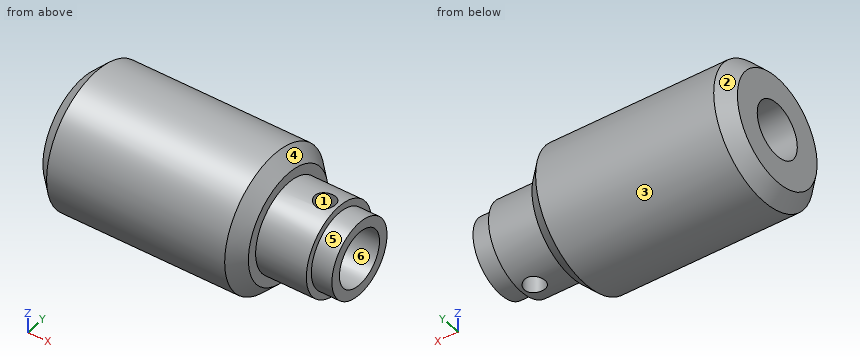
Autodesk Inventor part; units mm, degrees
ref_plane "Work Plane1" through (17.6, 0, -3.25) normal (0, 0, 1) x (1, 0, 0)
ref_plane "YZ Plane" through (0, 0, 0) normal (1, 0, 0) x (0, 1, 0)
ref_plane "XZ Plane" through (0, 0, 0) normal (0, 1, 0) x (-1, 0, 0)
sketch "Sketch1" plane through (0, 0, 0) normal (0, 0, 1) x (1, 0, 0)
  line L0 (0, 0) -> (0, 4.975)
  line L1 (0, 4.975) -> (15, 4.975)
  line L2 (15, 4.975) -> (15, 3.25)
  line L3 (15, 3.25) -> (20.2, 3.25)
  line L4 (20.2, 3.25) -> (20.2, 0)
  line L5 (20.2, 0) -> (0, 0)
  dimension "d2" = 20.2
  dimension "d3" = 15
  dimension "d19" = 9.95
  dimension "d20" = 6.5
revolve "Revolution1" add sketch "Sketch1" angle 360 about axis through (20.2, 0, 0) along (-1, 0, 0)
thread "Thread1"
chamfer "Chamfer1" distance 1 angle 45 2 edges at (15, -4.975, 0) (0, -4.975, 0)
hole "Hole1" at (20.2, 0, 0) direction (-1, 0, 0) diameter 4 end through all
ref_plane "Work Plane1" through (17.6, 0, -3.25) normal (0, 0, 1) x (1, 0, 0)
sketch "Sketch2" plane through (17.6, 0, -3.25) normal (0, 0, 1) x (1, 0, 0)
  line L0 (2.6, -3.25) -> (2.6, 3.25)
  line L1 (-2.6, -3.25) -> (-2.6, 3.25)
  point P0 (-17.6, 0)
  point P1 (0.1, 0)
  point P2 (2.6, 0)
  dimension "d21" = 2.5
hole "Hole2" at (17.7, 0, -3.25) direction (0, 0, 1) diameter 1.5 end through all
sketch "Sketch3" plane through (20.2, 0, 0) normal (1, 0, 0) x (0, 0, -1)
  circle A0 centre (0, 0) radius 2.75
  circle A1 centre (0, 0) radius 3.25
  dimension "d29" = 5.5
extrude "Extrusion1" cut sketch "Sketch3" against normal blind 1.5
properties part number "worm_1_20_conrad_with_bolt_hole" material "Steel"
Geometry: final body of the model. Coordinates: model frame, mm. Face numbers are marked on the shaded views. A direction names the side the tool comes from. Coordinates: 2 decimals unless noted, no trailing zeros. Order: outer loops, then holes, each group sorted by start corner. A loop starts at its lowest first (then second) coordinate and runs counter-clockwise, first axis right, second up.
Item 1: Access query for the marked faces 5 and 6. Directions: +Z, -Z, +X, -X, +Y, -Y. A direction counts if a zero-diameter tool reaches every point of the face in a straight line with its end or side. Return the directions, or none.
Answer:
face 5: +X
face 6: +X, -X
Item 2: Material intervals for line 1 along X through (y, z) = (0, -2.7); line 2 along Y through (x, z) = (8.75, 0) (3 decimals), sorted ascending.
Answer:
line 1: x = 0 to 16.95, 18.45 to 20.2
line 2: y = -4.975 to -2, 2 to 4.975
Item 3: Section query C-C (x = 4.75). Output: boundary loops of the cut face in (y, z) (3 decimals).
Answer:
outline: circle Ø9.95 at (0, 0); hole circle Ø4 at (0, 0)
Item 4: Section query B-B (x = 17.7). Output: boundary loops of the cut face in (y, z).
Answer:
outline: (-0.75, -3.16) - (-0.75, -1.85) arc R2 cw to (-0.75, 1.85) - (-0.75, 3.16) arc R3.25 ccw to start; (0.75, -3.16) arc R3.25 ccw to (0.75, 3.16) - (0.75, 1.85) arc R2 cw to (0.75, -1.85) - close
Item 5: Section query A-A (z = 0). Output: boundary loops of the cut face in (x, y) (3 decimals), then the cut area to 4 significant figures.
Answer:
outline: (0, -3.975) - (1, -4.975) - (14, -4.975) - (15, -3.975) - (15, -3.25) - (18.7, -3.25) - (18.7, -2.75) - (20.2, -2.75) - (20.2, -2) - (0, -2) - close; (0, 2) - (20.2, 2) - (20.2, 2.75) - (18.7, 2.75) - (18.7, 3.25) - (15, 3.25) - (15, 3.975) - (14, 4.975) - (1, 4.975) - (0, 3.975) - close
area: 98.75 mm2
Item 6: Contact query for flat-ended pins moving along their axis: P1, Ø2.5, axis at y = 0, z = 0, coming from the -X side; P2, Ø4, axis at x = 5, z = -2.5, coming from the +Y side; P3, Ø1.5, axis at x = 18, z = 2, coming from the +Y side; P4, Ø1.7, axis at x = 17.7, y = 0, coming from the -Z side. Output: stop coordinate, or through.
Answer:
P1: passes through
P2: stops at y = 4.95
P3: stops at y = 3
P4: stops at z = -3.25
Item 7: Draft query along X for the marked faces 1, 2, 3 and 4. Return one class per face: released by +X, released by -X, zero draft, split by the parting line, or undercut.
Answer:
face 1: undercut
face 2: released by -X
face 3: zero draft
face 4: released by +X
